Here's how the part is built. I have some questions about the finished solid (model axes, mm). Coordinates: 2 decimals unless noted, no trailing zeros. Loops run counter-clockwise (first coordinate to the right, second up) from the corner with the lowest first, then second, coordinate; pieces in that order, holes last. Notation, with made-up numbers: (64, 24) -> (104, 24) arc R10 cw to (104, 36) -> close; hole circle Ø7 at (6, 66.5). An arc over 180 degrees is marked (long way). Answer as a JSON object with one key per item and string values. Group by question number.
Q1. I want a section at A-A on z = -131.5. Write out the boundary of the cut face in (x, y).
Q2. I need wall thicknesses on line 1 (Y direction, x = 1.8, z = 0); line 2 (Z direction, x = 0.4, y = -117.5); line 3 (Y direction, x = 1.1, z = -126.5). Which ranges of each line are inside material? Lowest first, please.
Q3. I'm going to push flat-ended pins straight in: pin 1 (2.5 mm diameter, centred on y = -98, z = 0, fed in from +X); pin 2 (1.5 mm diameter, centred on x = 1, y = -105, fed in from +Z); pin 3 (0.9 mm diameter, centred on x = 2, z = 145.5, fed in from +Y); pin 4 (1.5 mm diameter, centred on x = 1, y = 147.5, fed in from -Z). Where does each tip first touch, or does it pass through?
Q4. I want a section at B-B on x = 0.6. Count the separate pieces of the cut face and the enclosed holes in it, then the cut area to 3 significant figures.
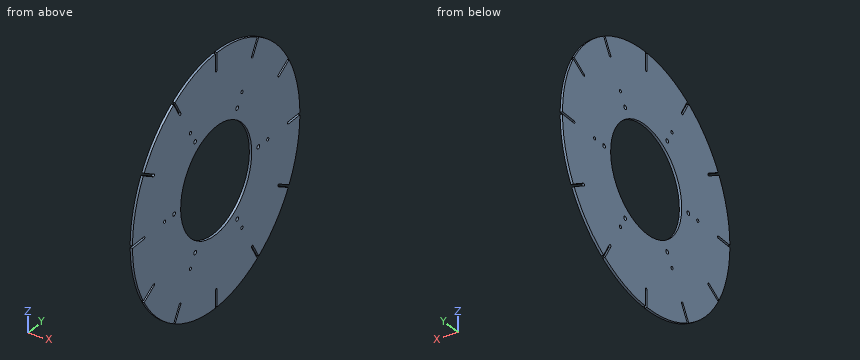
```python
from build123d import *

# Parameters (mm, degrees)
SKETCH1_R           = 159
BOSS_EXTRUDE1_DEPTH = 3
SKETCH2_R           = 2
SKETCH2_R_2         = 1.5
SKETCH2_R_3         = 2.5
SKETCH2_R_4         = 67.5
CUT_EXTRUDE1_DEPTH  = 3
CUT_EXTRUDE2_DEPTH  = 225.879967983
CIRPATTERN1_COUNT   = 12


with BuildPart() as part:
    # Sketch1 → Boss-Extrude1 (new body)
    with BuildSketch(Plane(origin=(0, 0, 0), x_dir=(0, 0, -1), z_dir=(1, 0, 0))):
        Circle(SKETCH1_R)
    extrude(amount=BOSS_EXTRUDE1_DEPTH)

    # Sketch2 → Cut-Extrude1 (cut)
    with BuildSketch(Plane(origin=(3, 0, 0), x_dir=(0, 0, -1), z_dir=(1, 0, 0))):
        with Locations((0, -98)):
            Circle(SKETCH2_R)
        with Locations((-84.870489571, -49)):
            Circle(SKETCH2_R)
        with Locations((-84.870489571, 49)):
            Circle(SKETCH2_R)
        with Locations((0, 98)):
            Circle(SKETCH2_R)
        with Locations((84.870489571, 49)):
            Circle(SKETCH2_R)
        with Locations((84.870489571, -49)):
            Circle(SKETCH2_R)
        with Locations((0, -150)):
            Circle(SKETCH2_R_2)
        with Locations((-129.903810568, -75)):
            Circle(SKETCH2_R_2)
        with Locations((-129.903810568, 75)):
            Circle(SKETCH2_R_2)
        with Locations((0, 150)):
            Circle(SKETCH2_R_2)
        with Locations((129.903810568, 75)):
            Circle(SKETCH2_R_2)
        with Locations((129.903810568, -75)):
            Circle(SKETCH2_R_2)
        with Locations((0, -80)):
            Circle(SKETCH2_R_3)
        with Locations((-69.282032303, -40)):
            Circle(SKETCH2_R_3)
        with Locations((-69.282032303, 40)):
            Circle(SKETCH2_R_3)
        with Locations((0, 80)):
            Circle(SKETCH2_R_3)
        with Locations((69.282032303, 40)):
            Circle(SKETCH2_R_3)
        with Locations((69.282032303, -40)):
            Circle(SKETCH2_R_3)
        Circle(SKETCH2_R_4)
    extrude(amount=-CUT_EXTRUDE1_DEPTH, mode=Mode.SUBTRACT)

    # Sketch3 → Cut-Extrude2 (cut, through all)
    with BuildSketch(Plane(origin=(3, 0, 0), x_dir=(0, 0, -1), z_dir=(1, 0, 0))):
        with BuildLine():
            Line((117.895480318, 69.799038106), (148.709562393, 87.589556686))
            ThreePointArc((148.709562393, 87.589556686), (150.758600499, 87.040518581), (150.209562393, 84.991480475))
            Line((150.209562393, 84.991480475), (119.395480318, 67.200961894))
            ThreePointArc((119.395480318, 67.200961894), (117.346442213, 67.75), (117.895480318, 69.799038106))
        make_face()
    cut_extrude2 = extrude(amount=-CUT_EXTRUDE2_DEPTH, mode=Mode.SUBTRACT)

    # CirPattern1: Cut-Extrude2 ×12 about axis
    cirpattern1_axis = Axis((0, 0, 0), (1, 0, 0))
    for i in range(1, CIRPATTERN1_COUNT):
        add(cut_extrude2.rotate(cirpattern1_axis, i * 360 / CIRPATTERN1_COUNT), mode=Mode.SUBTRACT)


solid = part.part
```
Result set:
{
 "1": {"outline": "(0, -89.38) -> (3, -89.38) -> (3, -77.65) -> (0, -77.65) -> close; (0, -74.19) -> (3, -74.19) -> (3, 74.19) -> (0, 74.19) -> close; (0, 77.65) -> (3, 77.65) -> (3, 89.38) -> (0, 89.38) -> close"},
 "2": {"line 1": "y = -135.5 to -100, -96 to -82.5, -77.5 to -67.5, 67.5 to 77.5, 82.5 to 96, 100 to 135.5", "line 2": "z = -107.12 to -69.47, -67.53 to 67.53, 69.47 to 107.12", "line 3": "y = -96.33 to -74.77, -71.3 to 71.3, 74.77 to 96.33"},
 "3": {"pin 1": "passes through", "pin 2": "stops at z = 120.05", "pin 3": "stops at y = 65.13", "pin 4": "stops at z = -61.2"},
 "4": {"separate pieces": "1", "enclosed holes": "13", "area": "64,100 mm²"}
}
